Input: part model. Units: mm. Frame: model coordinates. A direction names the side the tool comes from. Round coordinates to 2 decimals unless told otherwise and drop trailing zeros. Loops run counter-clockwise (first coordinate to the right, second up) from the corner with the lowest first, then second, coordinate; pieces in that order, holes last. Notation, with made-up numbers: (43, -26) -> (95, -26) arc R8 ccw to (95, -18) -> close; hole circle Ø5 at (22.5, 88). An arc over 180 degrees is marked (long way). One line per question, with ' | ' between items. Start each with the question number.
Q1. Cut plane C-C on x = 3.5. Return loops of the section in (y, z) (3 decimals), and give its area (3 significant figures).
Q2. Access query for faces 1 (the face through (10, -2, 8)), 2 (the face through (4, 27, 8)), 3 (the face through (-5, 12, 15)), 4 (the face through (-7, -6, 8)). Directions: +Z, -Z, +X, -X, +Y, -Y. A direction counts if a zero-diameter tool reaches every point of the face in a straight line with its end or side. Return the directions, or none.
Q3. Cut plane D-D on z = 1.5. Return loops of the section in (x, y).
Q4. Cut plane B-B on z = 8. Return loops of the section in (x, y), and give its area (3 significant figures).
Q5. Cut plane A-A on x = -1. Return loops of the section in (y, z).
Q6. Contact query for flat-ended pins moving along their axis: P1, Ø1, axis at y = 6, z = 15.5, coming from the +X side; P2, Ø1.8, axis at y = -6.5, z = 7, coming from the +X side; P3, Ø3, axis at x = 4.5, y = -6, coming from the -Z side; P4, Ø2.5, axis at x = -1, z = 8, coming from the -Y side. Output: stop coordinate, or through.
Q7. Mould query, pull axis X, two halves, no side actions, for faces 5 (the face through (-1.914, 29.187, 9.433)), 6 (the face through (2.4, 25.48, 14.99)), 7 (the face through (2, -3, 8)). Classes: pulls with the +X half, pulls with the -X half, needs draft (parallel to the pull), parting line crosses it, or undercut.
Q8. Material intervals for L1, parallel to Y at x = -4.5, z = 10; L2, parallel to X at y = 28.7, z = 8; L3, parallel to Z at x = -1, y = 29.15, sorted ascending.
from build123d import *

# Parameters (mm, degrees)
PAD_DEPTH        = 16
SKETCH001_W      = 27
SKETCH001_H      = 12
SKETCH001_W_2    = 7
POCKET_DEPTH     = 17
HOLE_D           = 3.4
HOLE_DEPTH       = 25
HOLE_CSINK_D     = 6.1
HOLE_CSINK_ANGLE = 90


with BuildPart() as part:
    # Sketch → Pad (new body)
    with BuildSketch(Plane.XY):
        Polygon((-10, -10), (10, -3), (10, 0), (-5, 0), (-5, 24), (10, 27), (10, 30), (-10, 30), align=None)
    extrude(amount=PAD_DEPTH)

    # Sketch001 (on Face6 of Pad) → Pocket (cut)
    with BuildSketch(Plane.YZ.offset(10)):
        with Locations((13.5, 8)):
            Rectangle(SKETCH001_W, SKETCH001_H)
        with Locations((-6.5, 8)):
            Rectangle(SKETCH001_W_2, SKETCH001_H)
    extrude(amount=-POCKET_DEPTH, mode=Mode.SUBTRACT)

    # Hole
    with Locations(Plane.XZ.offset(-27)):
        with Locations((-1, 8)):
            CounterSinkHole(HOLE_D / 2, HOLE_CSINK_D / 2, depth=HOLE_DEPTH, counter_sink_angle=HOLE_CSINK_ANGLE)


solid = part.part
Results:
1) outline: (-5.275, 0) -> (0, 0) -> (0, 16) -> (-5.275, 16) -> (-5.275, 14) -> (-3, 14) -> (-3, 2) -> (-5.275, 2) -> close; (25.7, 0) -> (30, 0) -> (30, 16) -> (25.7, 16) -> (25.7, 14) -> (27, 14) -> (27, 2) -> (25.7, 2) -> close | area: 110 mm^2
2) face 1: +Z, -Z, +X, +Y, -Y | face 2: +X | face 3: +Z, -Z, +X | face 4: +X, -Y
3) outline: (-10, -10) -> (10, -3) -> (10, 0) -> (-5, 0) -> (-5, 24) -> (10, 27) -> (10, 30) -> (-10, 30) -> close
4) outline: (-10, -10) -> (-7, -8.95) -> (-7, -3) -> (10, -3) -> (10, 0) -> (-7, 0) -> (-7, 27) -> (-4.05, 27) -> (-2.7, 28.35) -> (-2.7, 30) -> (-10, 30) -> close; (0.7, 28.35) -> (2.05, 27) -> (10, 27) -> (10, 30) -> (0.7, 30) -> close | area: 208 mm^2
5) outline: (-6.85, 0) -> (0, 0) -> (0, 16) -> (-6.85, 16) -> (-6.85, 14) -> (-3, 14) -> (-3, 2) -> (-6.85, 2) -> close; (24.8, 0) -> (30, 0) -> (30, 6.3) -> (28.35, 6.3) -> (27, 4.95) -> (27, 2) -> (24.8, 2) -> close; (24.8, 14) -> (27, 14) -> (27, 11.05) -> (28.35, 9.7) -> (30, 9.7) -> (30, 16) -> (24.8, 16) -> close
6) P1: x = -5 | P2: x = -7 | P3: z = 0 | P4: y = -3
7) face 5: undercut | face 6: pulls with the +X half | face 7: needs draft
8) L1: -3 to 0, 27 to 30 | L2: -10 to -2.7, 0.7 to 10 | L3: 0 to 6.3, 9.7 to 16
